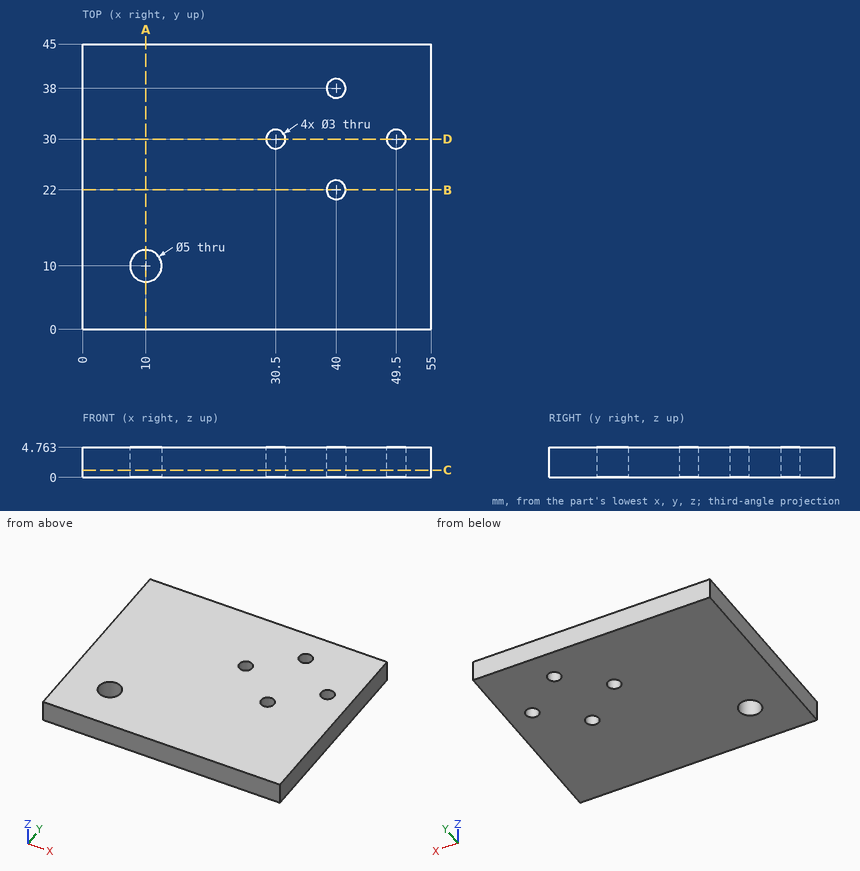
Source: three-view drawing plus pictorial views. Frame: mm from the lowest corner of the part. Give positions to 0.01 mm unless a question says otherwise; leave off trailing zeros. Loops run counter-clockwise (first coordinate to the right, second up) from the corner with the lowest first, then second, coordinate; pieces in that order, holes last.
1) Section query C-C on z = 1.15. Return the cut outline in (x, y), and give its area (3 significant figures).
A:
outline: (0, 0) - (55, 0) - (55, 45) - (0, 45) - close; hole circle Ø5 at (10, 10); hole circle Ø3 at (30.5, 30); hole circle Ø3 at (40, 22); hole circle Ø3 at (40, 38); hole circle Ø3 at (49.5, 30)
area: 2,430 mm2
2) Section query D-D on y = 30. Return the cut outline in (x, z), and give its area (3 significant figures).
A:
outline: (0, 0) - (29, 0) - (29, 4.76) - (0, 4.76) - close; (32, 0) - (48, 0) - (48, 4.76) - (32, 4.76) - close; (51, 0) - (55, 0) - (55, 4.76) - (51, 4.76) - close
area: 233 mm2
3) Section query A-A on x = 10. Return the cut outline in (y, z).
A:
outline: (0, 0) - (7.5, 0) - (7.5, 4.76) - (0, 4.76) - close; (12.5, 0) - (45, 0) - (45, 4.76) - (12.5, 4.76) - close
4) Section query B-B on y = 22. Return the cut outline in (x, z), and give its area (3 significant figures).
A:
outline: (0, 0) - (38.5, 0) - (38.5, 4.76) - (0, 4.76) - close; (41.5, 0) - (55, 0) - (55, 4.76) - (41.5, 4.76) - close
area: 248 mm2
5) Line query: L1, parallel to X at y = 30, z = 2.55; L2, parallel to Y at x = 40, z = 1.3; L3, parallel to X at y = 10, z = 1.3. Output: solid intervals per line, ascending.
A:
L1: x = 0 to 29, 32 to 48, 51 to 55
L2: y = 0 to 20.5, 23.5 to 36.5, 39.5 to 45
L3: x = 0 to 7.5, 12.5 to 55
